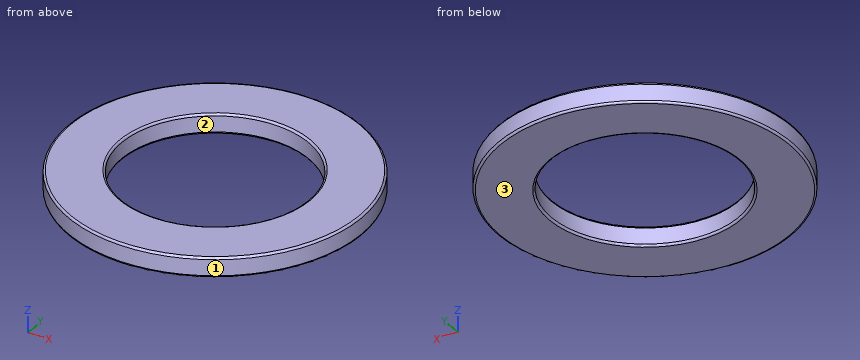
```python
from build123d import *

# Parameters (mm, degrees)
SKETCH1_R          = 11.075
SKETCH1_R_2        = 7.075
BASE_FLANGE1_DEPTH = 1.5
FILLET1_R          = 0.15


# Sheet-metal steps are written as plain solids
with BuildPart() as part:
    # Sketch1 → Base-Flange1 (new body)
    with BuildSketch(Plane.XY):
        Circle(SKETCH1_R)
        Circle(SKETCH1_R_2, mode=Mode.SUBTRACT)
    extrude(amount=-BASE_FLANGE1_DEPTH)

    # Fillet1
    fillet1_edges = [part.edges().sort_by_distance(p)[0] for p in [
        (-11.075, 0, 0),
        (-11.075, 0, -1.5),
        (-7.075, 0, -1.5),
        (-7.075, 0, 0),
    ]]
    fillet(fillet1_edges, radius=FILLET1_R)


solid = part.part
```
Verification items for the finished model (mm, model axes). Face numbers are marked on the shaded views. Coordinates: 2 decimals unless noted, no trailing zeros. Loops run counter-clockwise (first coordinate to the right, second up) from the corner with the lowest first, then second, coordinate; pieces in that order, holes last. Notation, with made-up numbers: (-0.5, 88.5) -> (24.5, 88.5) arc R14 cw to (24.5, 98.5) -> close; hole circle Ø11 at (17, -27). An arc over 180 degrees is marked (long way). Answer in a Markdown table with one row per item. Add a question column.
1. Section check A-A, the plane y = 0. Enter the section's corners in (x, z) (3 decimals).
2. Material ranges on probe 1 along Y at (x, z) = (0, -0.4) (3 decimals); probe 2 along Y at (x, z) = (2.5, -0.8); probe 3 along X at (y, z) = (0.5, -0.7), recorded low to high. Write a range as [from, to].
3. Depth check by flat-ended pin: P1, Ø12.5, axis at x = 0, y = 0, coming from the +Z side. Enter the tip coordinate at first touch or a pass-through.
4. Draft check along Y on the marked faces 1, 2 and 3. Enter one of: +Y half, -Y half, draft (parallel to the pull), parting line (faces both ways), or undercut.
5. Section check C-C, the plane z = -0.6. Enter the section's corners in (x, y) (3 decimals), then the cut area to 3 significant figures.
Derived:
| question | item | result |
|---|---|---|
| 1 | outline | (-11.075, -1.35) arc R0.15 ccw to (-10.925, -1.5) -> (-7.225, -1.5) arc R0.15 ccw to (-7.075, -1.35) -> (-7.075, -0.15) arc R0.15 ccw to (-7.225, 0) -> (-10.925, 0) arc R0.15 ccw to (-11.075, -0.15) -> close; (7.075, -1.35) arc R0.15 ccw to (7.225, -1.5) -> (10.925, -1.5) arc R0.15 ccw to (11.075, -1.35) -> (11.075, -0.15) arc R0.15 ccw to (10.925, 0) -> (7.225, 0) arc R0.15 ccw to (7.075, -0.15) -> close |
| 2 | probe 1 | y = [-11.075, -7.075], [7.075, 11.075] |
| 2 | probe 2 | y = [-10.79, -6.62], [6.62, 10.79] |
| 2 | probe 3 | x = [-11.06, -7.06], [7.06, 11.06] |
| 3 | P1 | passes through |
| 4 | face 1 | parting line |
| 4 | face 2 | undercut |
| 4 | face 3 | draft |
| 5 | outline | circle Ø22.15 at (0, 0); hole circle Ø14.15 at (0, 0) |
| 5 | area | 228 mm² |
